Geometry: final body of the model. Coordinates: model frame, mm. A direction names the side the tool comes from. Give positions to 0.01 mm unless a question says otherwise; leave off trailing zeros. Write each loop counter-clockwise with the first axis right and the second up, starting at its lowest first coordinate (ties: lowest second). Pieces come first, ordered by that corner, then holes. Notation, with made-up numbers: M 58,6 L 73,6 A29 ccw 73,31 Z; hole C 85.5,2 d1. An arc over 180 degrees is marked long. Use one line per item in the form item = value. Start each with the question number.
Item 1: Access query for faces 4 (the flat face through (-5, -11, 7)), 5 (the flat face through (-13, -11, 5)), 6 (the flat face through (3, -11, 2.5)), 7 (the flat face through (1, -20, 1)). Directions: +Z, -Z, +X, -X, +Y, -Y. A direction counts if a zero-diameter tool reaches every point of the face in a straight line with its end or side. Return the directions, or none.
Item 2: Contact query for flat-ended pins moving along their axis: P1, Ø2, axis at x = 6, z = 4.5, coming from the +Y side; P2, Ø3, axis at x = 0, z = 5, coming from the -Y side; P3, Ø2.5, axis at x = 1, y = -9.5, coming from the -Z side. Output: stop coordinate, or through.
Item 3: Section query C-C on z = 5.75. Return loops of the section in (x, y).
Item 4: Section query A-A on y = -13.25. Return loops of the section in (x, z).
Item 5: Section query B-B on x = -11.5. Return loops of the section in (y, z).
Item 6: Section query D-D on z = 1.5. Return loops of the section in (x, y), then the cut area to 3 significant figures.
Item 7: Material intervals for line 1 along X through (y, z) = (-11.75, 5.25); line 2 along X through (y, z) = (-14.5, 6.75); line 3 along Y through (x, z) = (-11.25, 3.5), sorted ascending. Write a range as from..to.
Item 8: Pull-direction query (X, two-part tool) for faces 1 (the flat face through (-7, -11, 6.5)), 2 (the flat face through (0.8, -21, 0.5)), 3 (the flat face through (16, -11, 4)); classes: released by +X, released by -X, zero draft, split by the parting line, or undercut.
from build123d import *

# Parameters (mm, degrees)
BOX038_W                   = 3
BOX038_H                   = 8
BOX038_DEPTH               = 4
BOX037_W                   = 8
BOX037_H                   = 8
BOX037_DEPTH               = 2
CHAMFER001_SIZE            = 1
CHAMFER001_PLACEMENT_ANGLE = 180
BOX004_W                   = 30
BOX004_H                   = 8
BOX004_DEPTH               = 2.5
BOX003_W                   = 30
BOX003_H                   = 15
BOX003_DEPTH               = 7.5
BOX002_W                   = 30
BOX002_H                   = 21
BOX002_DEPTH               = 1


with BuildPart() as cubo038:
    # Box038 → Box038 (new body)
    with BuildSketch(Plane(origin=(-13, -15, 2.5), x_dir=(1, 0, 0), z_dir=(0, 0, 1))):
        with Locations((1.5, 4)):
            Rectangle(BOX038_W, BOX038_H)
    extrude(amount=BOX038_DEPTH)


with BuildPart() as fusion002023:
    # Box037 → Box037 (new body)
    with BuildSketch(Plane(origin=(-13, -15, 6), x_dir=(1, 0, 0), z_dir=(0, 0, 1))):
        with Locations((4, 4)):
            Rectangle(BOX037_W, BOX037_H)
    extrude(amount=BOX037_DEPTH)

    # Chamfer001
    chamfer001_edges = [fusion002023.edges().sort_by_distance(p)[0] for p in [
        (-13, -11, 8),
    ]]
    chamfer(chamfer001_edges, length=CHAMFER001_SIZE)


with BuildPart() as fusion002023_1:
    # Chamfer001 placement: moved
    add(fusion002023.part.moved(Location((-18, -22, 0.5))).rotate(Axis((-18, -22, 0.5), (0, 0, 1)), CHAMFER001_PLACEMENT_ANGLE))

    # Fusion002023: union Cubo038
    add(cubo038.part)


with BuildPart() as cubo004:
    # Box004 → Box004 (new body)
    with BuildSketch(Plane(origin=(-14, -15, 0), x_dir=(1, 0, 0), z_dir=(0, 0, 1))):
        with Locations((15, 4)):
            Rectangle(BOX004_W, BOX004_H)
    extrude(amount=BOX004_DEPTH)


with BuildPart() as cubo003:
    # Box003 → Box003 (new body)
    with BuildSketch(Plane(origin=(-14, -18.5, 0), x_dir=(1, 0, 0), z_dir=(0, 0, 1))):
        with Locations((15, 7.5)):
            Rectangle(BOX003_W, BOX003_H)
    extrude(amount=BOX003_DEPTH)


with BuildPart() as cut059:
    # Box002 → Box002 (new body)
    with BuildSketch(Plane(origin=(-14, -21, 0), x_dir=(1, 0, 0), z_dir=(0, 0, 1))):
        with Locations((15, 10.5)):
            Rectangle(BOX002_W, BOX002_H)
    extrude(amount=BOX002_DEPTH)

    # Fusion001: union Cubo003
    add(cubo003.part)

    # Cut006: cut Cubo004
    add(cubo004.part, mode=Mode.SUBTRACT)

    # Cut059: cut Fusion002023
    add(fusion002023_1.part, mode=Mode.SUBTRACT)


solid = cut059.part
Answer sheet:
q1.face_4 = +Z
q1.face_5 = +Z, -Z
q1.face_6 = -Z, +X, -X
q1.face_7 = +Z, +X, -X, -Y
q2.P1 = -3.5
q2.P2 = -18.5
q2.P3 = 2.5
q3.outline = M -14,-18.5 L 16,-18.5 L 16,-3.5 L -14,-3.5 Z; hole M -13,-15 L -10,-15 L -10,-7 L -13,-7 Z
q4.outline = M -14,2.5 L -13,2.5 L -13,7.5 L -14,7.5 Z; M -10,2.5 L 16,2.5 L 16,7.5 L -5,7.5 L -5,6.5 L -10,6.5 Z
q5.outline = M -21,0 L -15,0 L -15,7.5 L -18.5,7.5 L -18.5,1 L -21,1 Z; M -7,0 L 0,0 L 0,1 L -3.5,1 L -3.5,7.5 L -7,7.5 Z
q6.outline = M -14,-18.5 L 16,-18.5 L 16,-15 L -14,-15 Z; M -14,-7 L 16,-7 L 16,-3.5 L -14,-3.5 Z
q6.area = 210 mm2
q7.line_1 = -14..-13, -10..16
q7.line_2 = -14..-13, -5..16
q7.line_3 = -18.5..-15, -7..-3.5
q8.face_1 = undercut
q8.face_2 = zero draft
q8.face_3 = released by +X
